```python
from build123d import *

# Parameters (mm, degrees)
SKETCH1_R                 = 49.657
BOSS_EXTRUDE1_DEPTH       = 6.35
CUT_EXTRUDE1_DEPTH        = 71.512111002
FILLET1_R                 = 6.35
FILLET2_R                 = 5.08
SKETCH4_R                 = 4.7625
CUT_EXTRUDE2_DEPTH        = 71.512111002
F_6_32_TAPPED_HOLE1_D     = 2.7051
F_6_32_TAPPED_HOLE1_DEPTH = 12.7
CIRPATTERN1_COUNT         = 6


with BuildPart() as part:
    # Sketch1 → Boss-Extrude1 (new body)
    with BuildSketch(Plane.XY):
        Circle(SKETCH1_R)
    extrude(amount=BOSS_EXTRUDE1_DEPTH)

    # Sketch3 → Cut-Extrude1 (cut, through all)
    with BuildSketch(Plane.XY.offset(6.35)):
        with BuildLine():
            Line((-3.81, 44.41388104), (-3.81, 26.192306699))
            ThreePointArc((-3.81, 26.192306699), (-9.518480656, 17.814850668), (-4.445, 9.038273032))
            Line((-4.445, 9.038273032), (-4.445, -9.038273032))
            ThreePointArc((-4.445, -9.038273032), (-9.518480656, -17.814850668), (-3.81, -26.192306699))
            Line((-3.81, -26.192306699), (-3.81, -44.41388104))
            ThreePointArc((-3.81, -44.41388104), (-44.577, 0), (-3.81, 44.41388104))
        make_face()
        with BuildLine():
            Line((3.81, 44.41388104), (3.81, 26.192306699))
            ThreePointArc((3.81, 26.192306699), (9.518480656, 17.814850668), (4.445, 9.038273032))
            Line((4.445, 9.038273032), (4.445, -9.038273032))
            ThreePointArc((4.445, -9.038273032), (9.518480656, -17.814850668), (3.81, -26.192306699))
            Line((3.81, -26.192306699), (3.81, -44.41388104))
            ThreePointArc((3.81, -44.41388104), (44.577, 0), (3.81, 44.41388104))
        make_face()
    extrude(amount=-CUT_EXTRUDE1_DEPTH, mode=Mode.SUBTRACT)

    # Fillet1
    fillet1_edges = [part.edges().sort_by_distance(p)[0] for p in [
        (-3.81, 44.41388104, 3.175),
        (-3.81, -44.41388104, 3.175),
        (3.81, 44.41388104, 3.175),
        (3.81, -44.41388104, 3.175),
    ]]
    fillet(fillet1_edges, radius=FILLET1_R)

    # Fillet2
    fillet2_edges = [part.edges().sort_by_distance(p)[0] for p in [
        (-3.81, 26.192306699, 3.175),
        (-4.445, 9.038273032, 3.175),
        (-4.445, -9.038273032, 3.175),
        (-3.81, -26.192306699, 3.175),
        (4.445, 9.038273032, 3.175),
        (3.81, 26.192306699, 3.175),
        (3.81, -26.192306699, 3.175),
        (4.445, -9.038273032, 3.175),
    ]]
    fillet(fillet2_edges, radius=FILLET2_R)

    # Sketch4 → Cut-Extrude2 (cut, through all)
    with BuildSketch(Plane.XY.offset(6.35)):
        with Locations((0, 17.4625)):
            Circle(SKETCH4_R)
        with Locations((0, -17.4625)):
            Circle(SKETCH4_R)
    extrude(amount=-CUT_EXTRUDE2_DEPTH, mode=Mode.SUBTRACT)

    # #6-32 Tapped Hole1
    with Locations(Plane(origin=(49.65699993, -0.002635703, 3.166396975), x_dir=(5.3078169e-05, 0.999999998591, 0), z_dir=(0.999999998591, -5.3078169e-05, 0))):
        with Locations((0, 0)):
            f_6_32_tapped_hole1 = Hole(F_6_32_TAPPED_HOLE1_D / 2, depth=F_6_32_TAPPED_HOLE1_DEPTH)

    # CirPattern1: #6-32 Tapped Hole1 ×6 about axis
    cirpattern1_axis = Axis((0, 0, 6.35), (0, 0, -1))
    for i in range(1, CIRPATTERN1_COUNT):
        add(f_6_32_tapped_hole1.rotate(cirpattern1_axis, i * 360 / CIRPATTERN1_COUNT), mode=Mode.SUBTRACT)


solid = part.part
```
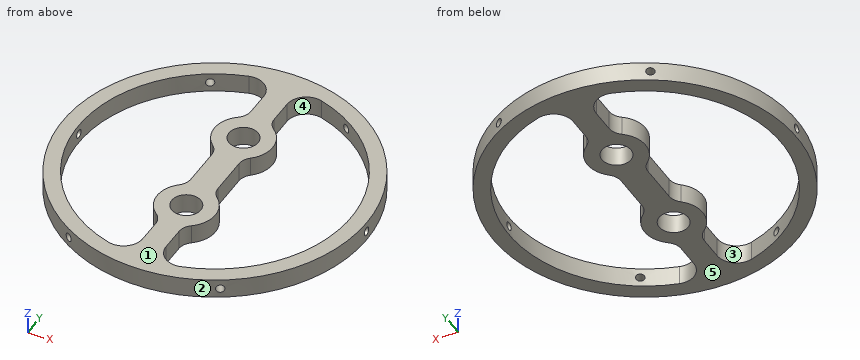
Source: CAD feature listing. Evaluate the final solid. Frame: model axes, mm. Face numbers are marked on the shaded views. A direction names the side the tool comes from. Round coordinates to 2 decimals unless told otherwise and drop trailing zeros. Order: outer loops, then holes, each group sorted by start corner. A loop starts at its lowest first (then second) coordinate and runs counter-clockwise, first axis right, second up. Notation, with made-up numbers: (37, -14) -> (71, -14) arc R25 ccw to (71, 8) -> close; hole circle Ø4 at (77, 10). An arc over 180 degrees is marked (long way). One line per item, written item: value. Start each with the question number.
Q1. Section query A-A (x = 0). Return the cut outline in (y, z) (3 decimals).
Q2. Access query for the marked faces 4 and 5. Directions: +Z, -Z, +X, -X, +Y, -Y. A direction counts if a zero-diameter tool reaches every point of the face in a straight line with its end or side. Return the directions, or none.
Q3. Section query D-D (y = -31). Return the cut outline in (x, z), plus the area to 3 significant figures.
Q4. Material intervals for probe 1 along Y at (x, z) = (0, 5) (3 decimals); probe 2 along X at (y, z) = (-17, 5.25); probe 3 along X at (y, z) = (-12.5, 5.5), sorted ascending.
Q5. Section query B-B (x = 15). Return the cut outline in (y, z), plus the area to 3 significant figures.
Q6. Section query C-C (y = -19.5). Return the cut outline in (x, z), plus the area to 3 significant figures.
Q7. Draft query along Y for the marked faces 1, 2 and 3. Return one class per face: pulls with the +Y half, pulls with the -Y half, needs draft (parallel to the pull), parting line crosses it, or undercut.
Q8. Pin query (flat end, axial travel): pin 1 (1.6 mm diameter, centred on y = 0, z = 3.17, fed in from +X) (3 decimals); pin 2 (3 mm diameter, centred on y = -34, z = 3, fed in from +X); pin 3 (3 mm diameter, centred on x = 35, z = 1.5, fed in from +Y). Return the tip coordinate at first contact, or that it passes through.
Findings below:
1. outline: (-49.657, 0) -> (-22.225, 0) -> (-22.225, 6.35) -> (-49.657, 6.35) -> close; (-12.7, 0) -> (12.7, 0) -> (12.7, 6.35) -> (-12.7, 6.35) -> close; (22.225, 0) -> (49.657, 0) -> (49.657, 6.35) -> (22.225, 6.35) -> close
2. face 4: +Z, -Z
2. face 5: -Z, +X, -X, +Y, -Y
3. outline: (-38.79, 0) -> (-32.03, 0) -> (-32.03, 6.35) -> (-38.79, 6.35) -> close; (-3.81, 0) -> (3.81, 0) -> (3.81, 6.35) -> (-3.81, 6.35) -> close; (32.03, 0) -> (38.79, 0) -> (38.79, 6.35) -> (32.03, 6.35) -> close
3. area: 134 mm²
4. probe 1: -49.657 to -22.225, -12.7 to 12.7, 22.225 to 49.657
4. probe 2: -46.66 to -41.21, -9.51 to -4.74, 4.74 to 9.51, 41.21 to 46.66
4. probe 3: -48.06 to -42.79, -8.13 to 8.13, 42.79 to 48.06
5. outline: (-47.34, 0) -> (-41.98, 0) -> (-41.98, 6.35) -> (-47.34, 6.35) -> close; (41.98, 0) -> (47.34, 0) -> (47.34, 6.35) -> (41.98, 6.35) -> close
5. area: 68.1 mm²
6. outline: (-45.67, 0) -> (-40.09, 0) -> (-40.09, 6.35) -> (-45.67, 6.35) -> close; (-9.3, 0) -> (-4.3, 0) -> (-4.3, 6.35) -> (-9.3, 6.35) -> close; (4.3, 0) -> (9.3, 0) -> (9.3, 6.35) -> (4.3, 6.35) -> close; (40.09, 0) -> (45.67, 0) -> (45.67, 6.35) -> (40.09, 6.35) -> close
6. area: 134 mm²
7. face 1: needs draft
7. face 2: parting line crosses it
7. face 3: undercut
8. pin 1: x = 4.445
8. pin 2: x = 37.54
8. pin 3: y = 36.65
